Can you work these out from the drawing? Everything is in mm from the part's minimum corner. Coordinates: 2 decimals unless noted, no trailing zeros. Loops run counter-clockwise (first coordinate to the right, second up) from the corner with the lowest first, then second, coordinate; pieces in that order, holes last. Notation, with made-up numbers: (35, -6) - (48, -6) arc R13 ccw to (48, 18) - close; hole circle Ø9 at (-1, 84.25). An arc over 180 degrees is marked (long way). One line per question, with ' | ' between items. Start each with the question number.
1. I want a section at C-C, the plane y = 8.41. Write out the boundary of the cut face in (x, z), then the cut area to 3 significant figures.
2. I want a section at B-B, the plane z = 18. Write out the boundary of the cut face in (x, y), then the cut area to 3 significant figures.
3. I want a section at D-D, the plane z = 2.75. Write out the boundary of the cut face in (x, y), then the cut area to 3 significant figures.
4. Please list where these lines run through material, in increasing order: L1, parallel to Z at x = 14.4, y = 12.5; L2, parallel to Y at x = 19.4, z = 3.75; L3, parallel to X at y = 9, z = 9.5. Write a range as [from, to].
5. I'm going to push flat-ended pins straight in: P1, Ø2.5, axis at x = 8, y = 8.5, coming from the -Z side; P2, Ø1.2, axis at x = 33.5, y = 8, coming from the -Z side. Where does each tip first touch, or does it pass through?
6. I want a section at A-A, the plane x = 14.4. Write out the boundary of the cut face in (y, z), then the cut area to 3 significant figures.
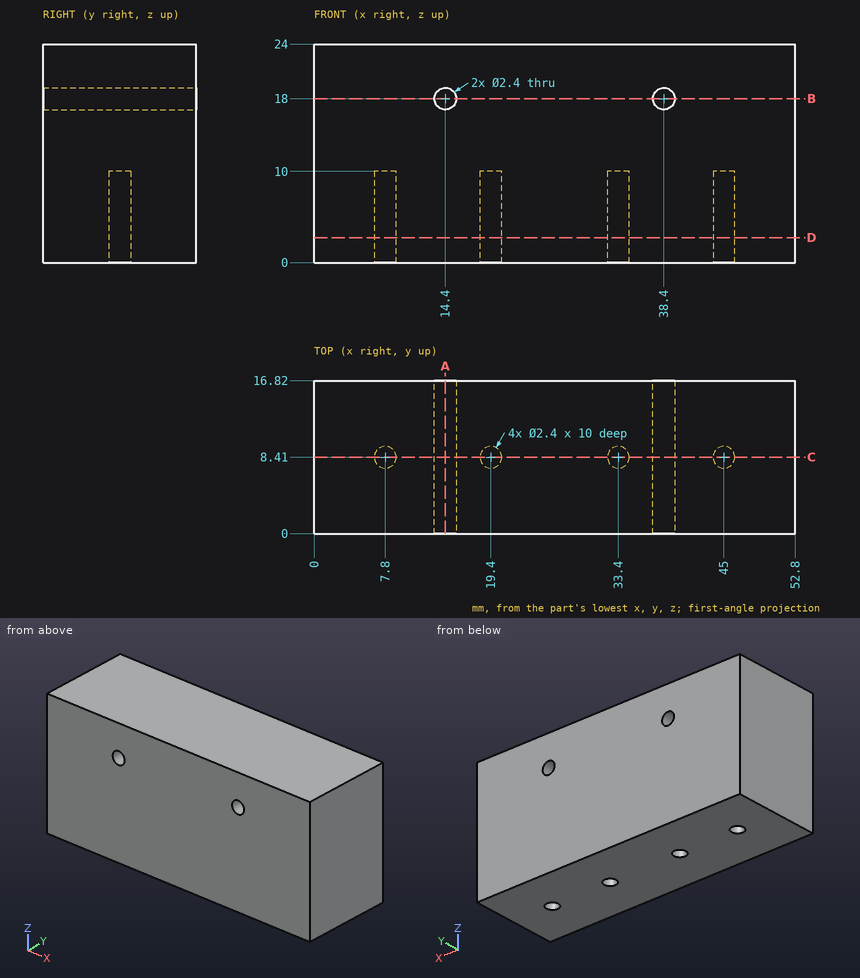
Results are:
1) outline: (0, 0) - (6.6, 0) - (6.6, 10) - (9, 10) - (9, 0) - (18.2, 0) - (18.2, 10) - (20.6, 10) - (20.6, 0) - (32.2, 0) - (32.2, 10) - (34.6, 10) - (34.6, 0) - (43.8, 0) - (43.8, 10) - (46.2, 10) - (46.2, 0) - (52.8, 0) - (52.8, 24) - (0, 24) - close; hole circle Ø2.4 at (14.4, 18); hole circle Ø2.4 at (38.4, 18) | area: 1,160 mm2
2) outline: (0, 0) - (13.2, 0) - (13.2, 16.82) - (0, 16.82) - close; (15.6, 0) - (37.2, 0) - (37.2, 16.82) - (15.6, 16.82) - close; (39.6, 0) - (52.8, 0) - (52.8, 16.82) - (39.6, 16.82) - close | area: 807 mm2
3) outline: (0, 0) - (52.8, 0) - (52.8, 16.82) - (0, 16.82) - close; hole circle Ø2.4 at (7.8, 8.41); hole circle Ø2.4 at (19.4, 8.41); hole circle Ø2.4 at (33.4, 8.41); hole circle Ø2.4 at (45, 8.41) | area: 870 mm2
4) L1: z = [0, 16.8], [19.2, 24] | L2: y = [0, 7.21], [9.61, 16.82] | L3: x = [0, 6.76], [8.84, 18.36], [20.44, 32.36], [34.44, 43.96], [46.04, 52.8]
5) P1: stops at z = 0 | P2: stops at z = 10
6) outline: (0, 0) - (16.82, 0) - (16.82, 16.8) - (0, 16.8) - close; (0, 19.2) - (16.82, 19.2) - (16.82, 24) - (0, 24) - close | area: 363 mm2
